Could you check a few things on this model? Use its own coordinates, in mm. Face numbers are marked on the shaded views. A direction names the side the tool comes from. Give positions to 0.01 mm unless a question says otherwise; leave off trailing zeros. Write each loop counter-clockwise with the first axis right and the second up, starting at its lowest first coordinate (ties: lowest second). Pieces come first, ordered by that corner, then holes. Notation, with made-up numbers: (22.25, -13.75) -> (52.25, -13.75) arc R9 ccw to (52.25, -6.75) -> close; hole circle Ø1 at (82, 65.5). An arc over 180 degrees is marked (long way). One line per question, with ' | ' between items.
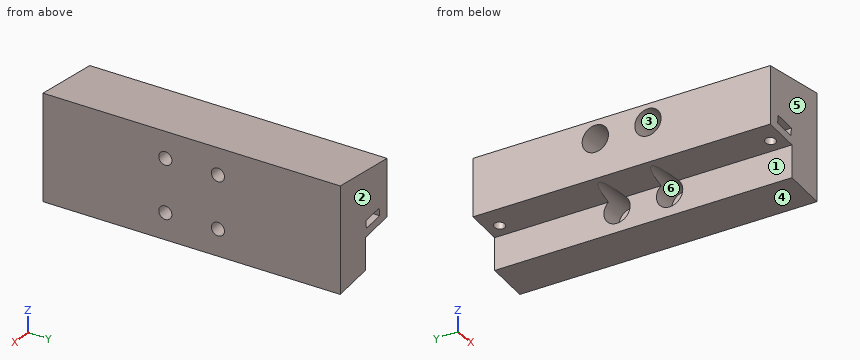
from build123d import *

# Parameters (mm, degrees)
BOSS_EXTRUDE1_DEPTH = 56.5
SKETCH2_R           = 2.5
CUT_EXTRUDE1_DEPTH  = 20
SKETCH5_R           = 5
CUT_EXTRUDE4_DEPTH  = 22
CUT_EXTRUDE5_DEPTH  = 126
SKETCH7_R           = 2
CUT_EXTRUDE6_DEPTH  = 6
CUT_EXTRUDE7_DEPTH  = 3
SKETCH10_R          = 2
CUT_EXTRUDE8_DEPTH  = 2


with BuildPart() as part:
    # Sketch1 → Boss-Extrude1 (new body, symmetric)
    with BuildSketch(Plane(origin=(0, 0, 0), x_dir=(1, 0, 0), z_dir=(0, 1, 0))):
        Polygon((0, 0), (-28, -3.175346835), (-28, -36.824653165), (0, -40), align=None)
    extrude(amount=BOSS_EXTRUDE1_DEPTH, both=True)

    # Sketch2 → Cut-Extrude1 (cut)
    with BuildSketch(Plane(origin=(0, 0, 0), x_dir=(0, 0, -1), z_dir=(1, 0, 0))):
        with Locations((-10, 10)):
            Circle(SKETCH2_R)
        with Locations((-10, -10)):
            Circle(SKETCH2_R)
        with Locations((-30, 10)):
            Circle(SKETCH2_R)
        with Locations((-30, -10)):
            Circle(SKETCH2_R)
    extrude(amount=-CUT_EXTRUDE1_DEPTH, mode=Mode.SUBTRACT)

    # Sketch5 → Cut-Extrude4 (cut)
    with BuildSketch(Plane.ZY.offset(28)):
        with Locations((30, 10)):
            Circle(SKETCH5_R)
        with Locations((30, -10)):
            Circle(SKETCH5_R)
        with Locations((10, -10)):
            Circle(SKETCH5_R)
        with Locations((10, 10)):
            Circle(SKETCH5_R)
    extrude(amount=-CUT_EXTRUDE4_DEPTH, mode=Mode.SUBTRACT)

    # Sketch6 → Cut-Extrude5 (cut)
    with BuildSketch(Plane.XZ.offset(56.5)):
        Polygon((-15, 1.701078662), (-15, 13.777996642), (-28, 15.252264816), (-28, 3.175346835), align=None)
    extrude(amount=-CUT_EXTRUDE5_DEPTH, mode=Mode.SUBTRACT)

    # Sketch7 → Cut-Extrude6 (cut)
    with BuildSketch(Plane(origin=(1.352195583, 0, 11.92357191), x_dir=(-0.993630993, 0, 0.112682965), z_dir=(-0.112682965, 0, -0.993630993))):
        with Locations((21.457010405, -51.5)):
            Circle(SKETCH7_R)
        with Locations((21.457010405, 51.5)):
            Circle(SKETCH7_R)
    extrude(amount=-CUT_EXTRUDE6_DEPTH, mode=Mode.SUBTRACT)

    # Sketch9 → Cut-Extrude7 (cut)
    with BuildSketch(Plane(origin=(2.028293375, 0, 17.885357866), x_dir=(-0.993630993, 0, 0.112682965), z_dir=(-0.112682965, 0, -0.993630993))):
        with BuildLine():
            Line((17.457010405, -51.5), (17.457010405, -56.5))
            Line((17.457010405, -56.5), (25.457010405, -56.5))
            Line((25.457010405, -56.5), (25.457010405, -51.5))
            ThreePointArc((25.457010405, -51.5), (21.457010405, -47.5), (17.457010405, -51.5))
        make_face()
        with BuildLine():
            Line((17.457010405, 56.5), (17.457010405, 51.5))
            ThreePointArc((17.457010405, 51.5), (21.457010405, 47.5), (25.457010405, 51.5))
            Line((25.457010405, 51.5), (25.457010405, 56.5))
            Line((25.457010405, 56.5), (17.457010405, 56.5))
        make_face()
    extrude(amount=CUT_EXTRUDE7_DEPTH, mode=Mode.SUBTRACT)

    # Sketch10 → Cut-Extrude8 (cut)
    with BuildSketch(Plane(origin=(2.028293375, 0, 17.885357866), x_dir=(-0.993630993, 0, 0.112682965), z_dir=(-0.112682965, 0, -0.993630993))):
        with Locations((21.457010405, 51.5)):
            Circle(SKETCH10_R)
        with Locations((21.457010405, -51.5)):
            Circle(SKETCH10_R)
    extrude(amount=-CUT_EXTRUDE8_DEPTH, mode=Mode.SUBTRACT)


solid = part.part
Q1. Imagine slicing it at B-B on z = 30. Please give me the cut outline in (x, y).
Answer below:
outline: (-28, -56.5) -> (0, -56.5) -> (0, -12.5) -> (-6, -12.5) -> (-6, -15) -> (-28, -15) -> close; (-28, -5) -> (-6, -5) -> (-6, -7.5) -> (0, -7.5) -> (0, 7.5) -> (-6, 7.5) -> (-6, 5) -> (-28, 5) -> close; (-28, 15) -> (-6, 15) -> (-6, 12.5) -> (0, 12.5) -> (0, 56.5) -> (-28, 56.5) -> close
Q2. Imagine slicing it at C-C on x = -8.5. Please give me the cut outline in (y, z).
Answer below:
outline: (-56.5, 0.96) -> (56.5, 0.96) -> (56.5, 39.04) -> (-56.5, 39.04) -> close; hole circle Ø10 at (-10, 10); hole circle Ø10 at (-10, 30); hole circle Ø10 at (10, 10); hole circle Ø10 at (10, 30)
Q3. On a 3-axis mill with a long thin cutter (end or side, diameter ignored), from which of +Z, -Z, +X, -X, +Y, -Y can I reach the whole of each face in a straight line? I mean the marked faces 1, 2 and 3. Say none if no direction works.
Answer below:
face 1: -Z, -X, +Y, -Y | face 2: +Z, -Z, +X, -X, +Y | face 3: -X
Q4. If I drill on line 1 along Y through (x, z) = (-15.5, 30); line 2 along Y through (x, z) = (-4.6, 10); line 3 along X through (y, z) = (-6.5, 8), over which ranges is the centre line in solid material (lowest first)?
Answer below:
line 1: y = -56.5 to -15, -5 to 5, 15 to 56.5 | line 2: y = -56.5 to -12.5, -7.5 to 7.5, 12.5 to 56.5 | line 3: x = -6 to 0
Q5. If we mould it in two halves opening along Y, with no side actions, what happens to the marked faces 4, 5 and 6? For each: +Y half, -Y half, draft (parallel to the pull), parting line (faces both ways), or undercut.
Answer below:
face 4: draft | face 5: -Y half | face 6: undercut
Q6. Will these pins go through, and if not, where does the flat tip stop? pin 1 (1.5 mm diameter, centred on x = -7, y = -5.5, fed in from -Z); pin 2 (5 mm diameter, centred on y = 12.5, z = 9.5, fed in from -X); pin 3 (5 mm diameter, centred on y = -10, z = 28.5, fed in from -X).
Answer below:
pin 1: stops at z = 0.71 | pin 2: stops at x = -15 | pin 3: stops at x = -6
Q7. Imagine slicing it at A-A on y = 10. Please give me the cut outline in (x, z).
Answer below:
outline: (-28, 15.25) -> (-25.78, 15) -> (-6, 15) -> (-6, 12.5) -> (0, 12.5) -> (0, 27.5) -> (-6, 27.5) -> (-6, 25) -> (-28, 25) -> close; (-28, 35) -> (-6, 35) -> (-6, 32.5) -> (0, 32.5) -> (0, 40) -> (-28, 36.82) -> close; (-15, 1.7) -> (0, 0) -> (0, 7.5) -> (-6, 7.5) -> (-6, 5) -> (-15, 5) -> close
Q8. Imagine slicing it at D-D on z = 6. Please give me the cut outline in (x, y).
Answer below:
outline: (-15, -56.5) -> (0, -56.5) -> (0, 56.5) -> (-15, 56.5) -> (-15, 13) -> (-6, 13) -> (-6, 7) -> (-15, 7) -> (-15, -7) -> (-6, -7) -> (-6, -13) -> (-15, -13) -> close
